Verification items for this drawing (mm, ordinates from the low corner). A direction names the side the tool comes from. Round coordinates to 2 decimals unless told otherwise and drop trailing zeros. Order: outer loops, then holes, each group sorted by start corner. A loop starts at its lowest first (then second) coordinate and runs counter-clockwise, first axis right, second up. Notation, with made-up numbers: (24, -29) - (57, -29) arc R22 ccw to (57, -1) - close; hole circle Ø1 at (-23, -5.75). An arc over 180 degrees is marked (long way). Return JSON: item names as keys, results as strings. Group by question number.
Q1. Sectioned sample at D-D, the plane y = 9.75. Record the cut outline in (x, z).
Q2. Sectioned sample at A-A, the plane z = 14.9. Record the cut outline in (x, y) (3 decimals), then the cut area to 3 significant figures.
Q3. Sectioned sample at C-C, the plane x = 3.25. Record the cut outline in (y, z) (3 decimals).
Q4. Gauge pin test, flat ends, axial feed: pin 1 Ø6 at (x, z) = (5.5, 7) entering from +Y; pin 2 Ø1 at (x, z) = (12.5, 17.5) entering from +Y; pin 3 Ø5 at (x, y) = (14, 18) entering from -Z. Record the tip position at first contact, or that the pin passes through.
Q5. Material ranges on line 1 along Y through (x, z) = (2.5, 15); line 2 along Z through (x, y) = (5.75, 14.9) (3 decimals); line 3 along Z through (x, y) = (14.5, 14.9) (3 decimals), recorded low to high.
Q6. Tool access check on the marked faces 4, 5 and 6. Record the directions out of +Z, -Z, +X, -X, +Y, -Y that give a thin tool (end or side, any length) a straight path to the whole face; none if there is none.
Q7. Draft check along Z on the marked faces 1, 2 and 3. Enter one of: pulls with the +Z half, pulls with the -Z half, needs draft (parallel to the pull), parting line crosses it, or undercut.
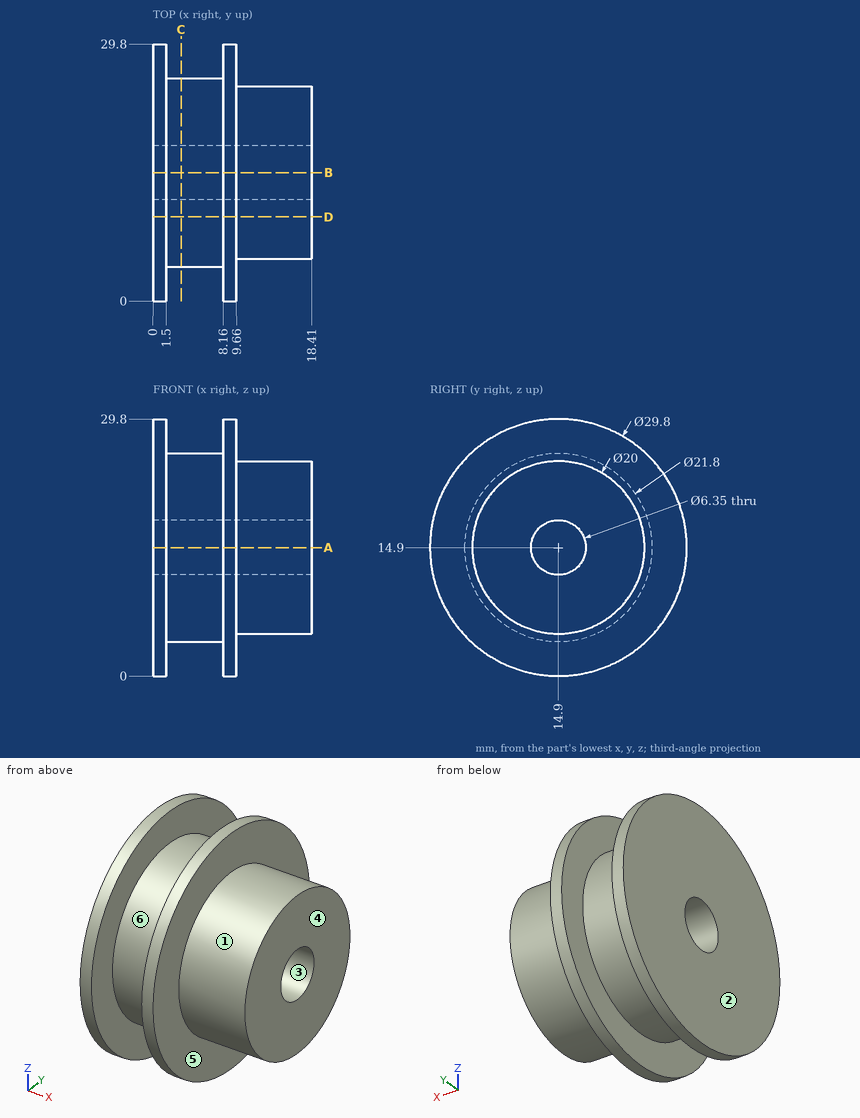
Reply:
{
 "1": {"outline": "(0, 0.92) - (1.5, 0.92) - (1.5, 5.29) - (8.16, 5.29) - (8.16, 0.92) - (9.66, 0.92) - (9.66, 6.33) - (18.41, 6.33) - (18.41, 23.47) - (9.66, 23.47) - (9.66, 28.88) - (8.16, 28.88) - (8.16, 24.51) - (1.5, 24.51) - (1.5, 28.88) - (0, 28.88) - close"},
 "2": {"outline": "(0, 0) - (1.5, 0) - (1.5, 4) - (8.16, 4) - (8.16, 0) - (9.66, 0) - (9.66, 4.9) - (18.41, 4.9) - (18.41, 11.725) - (0, 11.725) - close; (0, 18.075) - (18.41, 18.075) - (18.41, 24.9) - (9.66, 24.9) - (9.66, 29.8) - (8.16, 29.8) - (8.16, 25.8) - (1.5, 25.8) - (1.5, 29.8) - (0, 29.8) - close", "area": "293 mm^2"},
 "3": {"outline": "circle Ø21.8 at (14.9, 14.9); hole circle Ø6.35 at (14.9, 14.9)"},
 "4": {"pin 1": "y = 28.3", "pin 2": "y = 24.68", "pin 3": "z = 4.92"},
 "5": {"line 1": "4 to 11.73, 18.07 to 25.8", "line 2": "4 to 11.725, 18.075 to 25.8", "line 3": "4.9 to 11.725, 18.075 to 24.9"},
 "6": {"face 4": "+Z, -Z, +X, +Y, -Y", "face 5": "+X", "face 6": "none"},
 "7": {"face 1": "parting line crosses it", "face 2": "needs draft", "face 3": "undercut"}
}
